Part model, mm, in its own coordinate system. A direction names the side the tool comes from. Coordinates: 2 decimals unless noted, no trailing zeros. Order: outer loops, then holes, each group sorted by start corner. A loop starts at its lowest first (then second) coordinate and runs counter-clockwise, first axis right, second up.
from build123d import *

# Parameters (mm, degrees)
BOSS_EXTRUDE1_DEPTH = 99.5
SKETCH3_R           = 1.45
CUT_EXTRUDE1_DEPTH  = 2


with BuildPart() as part:
    # Sketch1 → Boss-Extrude1 (new body)
    with BuildSketch(Plane.XY):
        with BuildLine():
            Line((-43.109449142, 21.05), (-40.071600604, 21.05))
            ThreePointArc((-40.071600604, 21.05), (-36.198793003, 27.718621574), (-28.95, 30.35))
            Line((-28.95, 30.35), (28.95, 30.35))
            ThreePointArc((28.95, 30.35), (36.198793003, 27.718621574), (40.071600604, 21.05))
            Line((40.071600604, 21.05), (43.109449142, 21.05))
            ThreePointArc((43.109449142, 21.05), (38.327899552, 29.845600956), (28.95, 33.35))
            Line((28.95, 33.35), (-28.95, 33.35))
            ThreePointArc((-28.95, 33.35), (-38.327899552, 29.845600956), (-43.109449142, 21.05))
        make_face()
        with BuildLine():
            Line((-43.25, 19.05), (-40.25, 19.05))
            ThreePointArc((-40.25, 19.05), (-40.205311787, 20.053970411), (-40.071600604, 21.05))
            Line((-40.071600604, 21.05), (-43.109449142, 21.05))
            ThreePointArc((-43.109449142, 21.05), (-43.214819009, 20.052466277), (-43.25, 19.05))
        make_face()
        with BuildLine():
            Line((-50.25, 19.05), (-43.25, 19.05))
            ThreePointArc((-43.25, 19.05), (-43.214819009, 20.052466277), (-43.109449142, 21.05))
            Line((-43.109449142, 21.05), (-54.071600604, 21.05))
            Line((-54.071600604, 21.05), (-54.071600604, 19.05))
            Line((-54.071600604, 19.05), (-50.25, 19.05))
        make_face()
        with BuildLine():
            ThreePointArc((40.071600604, 21.05), (40.205311787, 20.053970411), (40.25, 19.05))
            Line((40.25, 19.05), (43.25, 19.05))
            ThreePointArc((43.25, 19.05), (43.214819009, 20.052466277), (43.109449142, 21.05))
            Line((43.109449142, 21.05), (40.071600604, 21.05))
        make_face()
        with BuildLine():
            ThreePointArc((43.109449142, 21.05), (43.214819009, 20.052466277), (43.25, 19.05))
            Line((43.25, 19.05), (50.25, 19.05))
            Line((50.25, 19.05), (54.071600604, 19.05))
            Line((54.071600604, 19.05), (54.071600604, 21.05))
            Line((54.071600604, 21.05), (43.109449142, 21.05))
        make_face()
    extrude(amount=BOSS_EXTRUDE1_DEPTH)

    # Sketch3 → Cut-Extrude1 (cut)
    with BuildSketch(Plane.XZ.offset(-19.05)):
        with Locations((-48.25, 79.5)):
            Circle(SKETCH3_R)
        with Locations((48.25, 20)):
            Circle(SKETCH3_R)
    extrude(amount=-CUT_EXTRUDE1_DEPTH, mode=Mode.SUBTRACT)


solid = part.part
Q1. Cut at B-B on z = 20. Write the cut outline in (x, y), and give its area (3 significant figures).
Results list:
outline: (-54.07, 19.05) - (-40.25, 19.05) arc R11.3 cw to (-28.95, 30.35) - (28.95, 30.35) arc R11.3 cw to (40.25, 19.05) - (46.8, 19.05) - (46.8, 21.05) - (43.11, 21.05) arc R14.3 ccw to (28.95, 33.35) - (-28.95, 33.35) arc R14.3 ccw to (-43.11, 21.05) - (-54.07, 21.05) - close; (49.7, 19.05) - (54.07, 19.05) - (54.07, 21.05) - (49.7, 21.05) - close
area: 332 mm2
Q2. Cut at D-D on z = 73. Write the cut outline in (x, y).
Results list:
outline: (-54.07, 19.05) - (-40.25, 19.05) arc R11.3 cw to (-28.95, 30.35) - (28.95, 30.35) arc R11.3 cw to (40.25, 19.05) - (54.07, 19.05) - (54.07, 21.05) - (43.11, 21.05) arc R14.3 ccw to (28.95, 33.35) - (-28.95, 33.35) arc R14.3 ccw to (-43.11, 21.05) - (-54.07, 21.05) - close
Q3. Mould opens along X. For faces 4 (the face through (47.1, 20.04, 19.12)), 5 (the face through (0, 30.35, 49)), 6 (the face through (38.436, 29.751, 49.054)), 7 (the face through (47, 19.05, 49)) say: pulls with the +X half, pulls with the -X half, needs draft (parallel to the pull), parting line crosses it, or undercut.
Results list:
face 4: undercut
face 5: undercut
face 6: pulls with the +X half
face 7: needs draft
Q4. Wall check: line 1 along Z through (x, y) = (48.25, 20.1); line 2 along X through (y, z) = (19.55, 79.5); line 3 along Z through (x, y) = (-48.25, 20.6). Give the ranges that are in metal, low to high.
Results list:
line 1: z = 0 to 18.55, 21.45 to 99.5
line 2: x = -54.07 to -49.7, -46.8 to -40.24, 40.24 to 54.07
line 3: z = 0 to 78.05, 80.95 to 99.5
Q5. Cut at C-C on y = 23.5. Write the cut outline in (x, z), and give its area (3 significant figures).
Results list:
outline: (-42.54, 0) - (-39.34, 0) - (-39.34, 99.5) - (-42.54, 99.5) - close; (39.34, 0) - (42.54, 0) - (42.54, 99.5) - (39.34, 99.5) - close
area: 637 mm2
Q6. Which spindle directions (+Z, -Z, +X, -X, +Y, -Y) get a long thin tool onto all of the face, cutting with end or side? Do faces 1 (the face through (-49, 21.05, 49)), 2 (the face through (49, 21.05, 49)), 3 (the face through (0, 33.35, 49)). Say none if no direction does.
Results list:
face 1: +Z, -Z, -X, +Y
face 2: +Z, -Z, +X, +Y
face 3: +Z, -Z, +X, -X, +Y
Q7. Pin check, flat tips, straight feed: pin 1 Ø9 at (x, z) = (-50, 26.5) entering from +Y; pin 2 Ø1 at (y, z) = (23.5, 87) entering from +X; pin 3 Ø8 at (x, y) = (38, 28.5) entering from -Z; pin 4 Ø10 at (x, z) = (-28.5, 34.5) entering from -Y. Stop position of each tip, or through.
Results list:
pin 1: stops at y = 21.05
pin 2: stops at x = 42.69
pin 3: stops at z = 0
pin 4: stops at y = 29.39
Q8. Cut at A-A on x = -48.25. Write the cut outline in (y, z), and give its area (3 significant figures).
Results list:
outline: (19.05, 0) - (21.05, 0) - (21.05, 78.05) - (19.05, 78.05) - close; (19.05, 80.95) - (21.05, 80.95) - (21.05, 99.5) - (19.05, 99.5) - close
area: 193 mm2
